from build123d import *

# Parameters (mm, degrees)
SKETCH1_W                 = 33
SKETCH1_H                 = 28
SKETCH1_R                 = 0.75
BOSS_EXTRUDE1_DEPTH       = 1.5
SKETCH2_W                 = 13
SKETCH2_H                 = 10
BOSS_EXTRUDE2_DEPTH       = 6.3
SKETCH3_W                 = 12
SKETCH3_H                 = 5.3
CUT_EXTRUDE1_DEPTH        = 9.5
CUT_EXTRUDE2_REACH        = 25.31
SKETCH5_W                 = 11
SKETCH5_H                 = 2
BOSS_EXTRUDE3_DEPTH       = 9.5
CHAMFER1_SIZE             = 1
CHAMFER1_SIZE2            = 1.804047755
CHAMFER1_OF_MIRROR4_SIZE2 = 1
CHAMFER1_OF_MIRROR4_SIZE  = 1.804047755


with BuildPart() as part:
    # Sketch1 → Boss-Extrude1 (new body)
    with BuildSketch(Plane(origin=(0, 0, 0), x_dir=(1, 0, 0), z_dir=(0, 1, 0))):
        Rectangle(SKETCH1_W, SKETCH1_H)
        with Locations(Location((-13.95, 11.5, 0), (0, 0, 270))):
            Circle(SKETCH1_R, mode=Mode.SUBTRACT)
        with Locations(Location((13.95, 11.5, 0), (0, 0, 270))):
            Circle(SKETCH1_R, mode=Mode.SUBTRACT)
        with Locations(Location((13.95, -1.7, 0), (0, 0, 270))):
            Circle(SKETCH1_R, mode=Mode.SUBTRACT)
        with Locations(Location((-13.95, -1.7, 0), (0, 0, 270))):
            Circle(SKETCH1_R, mode=Mode.SUBTRACT)
    extrude(amount=BOSS_EXTRUDE1_DEPTH)

    # Sketch2 → Boss-Extrude2 (add)
    with BuildSketch(Plane(origin=(0, 1.5, 0), x_dir=(1, 0, 0), z_dir=(0, 1, 0))):
        with Locations((-8.1, -9.5)):
            Rectangle(SKETCH2_W, SKETCH2_H)
    boss_extrude2 = extrude(amount=BOSS_EXTRUDE2_DEPTH)

    # Sketch3 → Cut-Extrude1 (cut)
    with BuildSketch(Plane.XY.offset(14.5)):
        with Locations((-8.1, 4.65)):
            Rectangle(SKETCH3_W, SKETCH3_H)
    cut_extrude1 = extrude(amount=-CUT_EXTRUDE1_DEPTH, mode=Mode.SUBTRACT)

    # Sketch4 → Cut-Extrude2 (cut, up to next)
    with BuildSketch(Plane(origin=(0, 7.8, 0), x_dir=(1, 0, 0), z_dir=(0, 1, 0)), mode=Mode.PRIVATE) as cut_extrude2_sk1:
        with BuildLine():
            Line((-13.614934874, -7.733680754), (-13.022262005, -10.296990911))
            ThreePointArc((-13.022262005, -10.296990911), (-13.006856344, -10.386514555), (-13.001698958, -10.477207547))
            Line((-13.001698958, -10.477207547), (-13.001698958, -11.69747768))
            ThreePointArc((-13.001698958, -11.69747768), (-12.650227096, -12.546005817), (-11.801698958, -12.89747768))
            Line((-11.801698958, -12.89747768), (-10.586140238, -12.89747768))
            ThreePointArc((-10.586140238, -12.89747768), (-9.7376121, -12.546005817), (-9.386140238, -11.69747768))
            Line((-9.386140238, -11.69747768), (-9.386140238, -10.477207547))
            ThreePointArc((-9.386140238, -10.477207547), (-9.380982852, -10.386514555), (-9.365577191, -10.296990911))
            Line((-9.365577191, -10.296990911), (-8.772904322, -7.733680754))
            ThreePointArc((-8.772904322, -7.733680754), (-8.922709401, -7.493767357), (-9.162622799, -7.643572436))
            Line((-9.162622799, -7.643572436), (-9.755295667, -10.206882592))
            ThreePointArc((-9.755295667, -10.206882592), (-9.778404159, -10.34116806), (-9.786140238, -10.477207547))
            Line((-9.786140238, -10.477207547), (-9.786140238, -11.69747768))
            ThreePointArc((-9.786140238, -11.69747768), (-10.020454813, -12.263163104), (-10.586140238, -12.49747768))
            Line((-10.586140238, -12.49747768), (-11.801698958, -12.49747768))
            ThreePointArc((-11.801698958, -12.49747768), (-12.367384383, -12.263163104), (-12.601698958, -11.69747768))
            Line((-12.601698958, -11.69747768), (-12.601698958, -10.477207547))
            ThreePointArc((-12.601698958, -10.477207547), (-12.609435037, -10.34116806), (-12.632543529, -10.206882592))
            Line((-12.632543529, -10.206882592), (-13.225216397, -7.643572436))
            ThreePointArc((-13.225216397, -7.643572436), (-13.465129794, -7.493767357), (-13.614934874, -7.733680754))
        make_face()
    cut_extrude2_tool1 = extrude(cut_extrude2_sk1.sketch, amount=-CUT_EXTRUDE2_REACH, mode=Mode.PRIVATE) & part.part
    # Sketch4 → Cut-Extrude2 (cut, up to next)
    with BuildSketch(Plane(origin=(0, 7.8, 0), x_dir=(1, 0, 0), z_dir=(0, 1, 0)), mode=Mode.PRIVATE) as cut_extrude2_sk2:
        with BuildLine():
            Line((-7.037377201, -7.643572436), (-6.444704333, -10.206882592))
            ThreePointArc((-6.444704333, -10.206882592), (-6.421595841, -10.34116806), (-6.413859762, -10.477207547))
            Line((-6.413859762, -10.477207547), (-6.413859762, -11.69747768))
            ThreePointArc((-6.413859762, -11.69747768), (-6.179545187, -12.263163104), (-5.613859762, -12.49747768))
            Line((-5.613859762, -12.49747768), (-4.398301042, -12.49747768))
            ThreePointArc((-4.398301042, -12.49747768), (-3.832615617, -12.263163104), (-3.598301042, -11.69747768))
            Line((-3.598301042, -11.69747768), (-3.598301042, -10.477207547))
            ThreePointArc((-3.598301042, -10.477207547), (-3.590564963, -10.34116806), (-3.567456471, -10.206882592))
            Line((-3.567456471, -10.206882592), (-2.974783603, -7.643572436))
            ThreePointArc((-2.974783603, -7.643572436), (-2.734870206, -7.493767357), (-2.585065126, -7.733680754))
            Line((-2.585065126, -7.733680754), (-3.177737995, -10.296990911))
            ThreePointArc((-3.177737995, -10.296990911), (-3.193143656, -10.386514555), (-3.198301042, -10.477207547))
            Line((-3.198301042, -10.477207547), (-3.198301042, -11.69747768))
            ThreePointArc((-3.198301042, -11.69747768), (-3.549772904, -12.546005817), (-4.398301042, -12.89747768))
            Line((-4.398301042, -12.89747768), (-5.613859762, -12.89747768))
            ThreePointArc((-5.613859762, -12.89747768), (-6.4623879, -12.546005817), (-6.813859762, -11.69747768))
            Line((-6.813859762, -11.69747768), (-6.813859762, -10.477207547))
            ThreePointArc((-6.813859762, -10.477207547), (-6.819017148, -10.386514555), (-6.834422809, -10.296990911))
            Line((-6.834422809, -10.296990911), (-7.427095678, -7.733680754))
            ThreePointArc((-7.427095678, -7.733680754), (-7.277290599, -7.493767357), (-7.037377201, -7.643572436))
        make_face()
    cut_extrude2_tool2 = extrude(cut_extrude2_sk2.sketch, amount=-CUT_EXTRUDE2_REACH, mode=Mode.PRIVATE) & part.part
    cut_extrude2_1 = cut_extrude2_tool1.solids().sort_by_distance((-13.247802, 7.8, 8.998967))[0]
    add(cut_extrude2_1, mode=Mode.SUBTRACT)
    cut_extrude2_2 = cut_extrude2_tool2.solids().sort_by_distance((-6.741196, 7.8, 11.087343))[0]
    add(cut_extrude2_2, mode=Mode.SUBTRACT)
    cut_extrude2 = cut_extrude2_1 + cut_extrude2_2  # Cut-Extrude2 as one shape, for the pattern or mirror that repeats it

    # Sketch5 → Boss-Extrude3 (add)
    with BuildSketch(Plane.XY.offset(5)):
        with Locations((-8.1, 5.8)):
            Rectangle(SKETCH5_W, SKETCH5_H)
    boss_extrude3 = extrude(amount=BOSS_EXTRUDE3_DEPTH)

    # Chamfer1
    chamfer1_edges = [part.edges().sort_by_distance(p)[0] for p in [
        (-8.1, 6.8, 14.5),
    ]]
    chamfer1_side = [part.faces().sort_by_distance(p)[0] for p in [
        (-8.1, 5.8, 14.5),
    ]]
    chamfer(chamfer1_edges, length=CHAMFER1_SIZE, length2=CHAMFER1_SIZE2, reference=chamfer1_side[0])

    # Mirror4: Boss-Extrude2, Cut-Extrude1, Cut-Extrude2, Boss-Extrude3 across plane
    add(boss_extrude2.mirror(Plane(origin=(0, 0, 0), x_dir=(0, 0, 1), z_dir=(1, 0, 0))))
    add(cut_extrude1.mirror(Plane(origin=(0, 0, 0), x_dir=(0, 0, 1), z_dir=(1, 0, 0))), mode=Mode.SUBTRACT)
    add(cut_extrude2.mirror(Plane(origin=(0, 0, 0), x_dir=(0, 0, 1), z_dir=(1, 0, 0))), mode=Mode.SUBTRACT)
    add(boss_extrude3.mirror(Plane(origin=(0, 0, 0), x_dir=(0, 0, 1), z_dir=(1, 0, 0))))

    # Chamfer1 of Mirror4
    chamfer1_of_mirror4_edges = [part.edges().sort_by_distance(p)[0] for p in [
        (8.1, 6.8, 14.5),
    ]]
    chamfer(chamfer1_of_mirror4_edges, length=CHAMFER1_OF_MIRROR4_SIZE, length2=CHAMFER1_OF_MIRROR4_SIZE2)


solid = part.part
Geometry: final body of the model. Coordinates: model frame, mm. A direction names the side the tool comes from. Give positions to 0.01 mm unless a question says otherwise; leave off trailing zeros. Write each loop counter-clockwise with the first axis right and the second up, starting at its lowest first coordinate (ties: lowest second). Pieces come first, ordered by that corner, then holes. Notation, with made-up numbers: (-21.5, 88.25) - (14.5, 88.25) arc R23 cw to (14.5, 120.25) - close; hole circle Ø7 at (27, -37.75). An arc over 180 degrees is marked (long way). Return JSON: item names as keys, results as strings. Group by question number.
1) Set-up query: faces 4 (the flat face through (8, 2, 10)), 5 (the flat face through (0, 1, 14)), 6 (the flat face through (14.6, 5, 10)), 7 (the cylindrical face through (9.75, 7.55, 12.56)), 8 (the flat face through (-14.6, 5, 10)). Return all of +Z, -Z, +X, -X, +Y, -Y with unobstructed straight access to the full face (end or side cutting, diameter ignored); none if empty.
2) Section D-D on z = 1.7. Return the cut outline in (x, y), plus the area to 3 significant figures.
3) Section C-C on y = 4. Return the cut outline in (x, z).
4) Section A-A on x = 11. Return the cut outline in (y, z).
5) Section B-B on y = 1. Return the cut outline in (x, z), plus the area to 3 significant figures.
6) First-contact query: P1, Ø1, axis at x = 0, z = -8, coming from the +Y side; P2, Ø0.5, axis at y = 7.5, z = 11, coming from the +X side; P3, Ø1, axis at x = 6.5, y = 4, coming from the -Z side. Flat tips, straight axial feed; report the tip coordinate or a pass-through.
7) Line query: line 1 (X direction, y = 4.75, z = 7.5); line 2 (Y direction, x = -8.5, z = 8.25); line 3 (X direction, y = 0.65, z = -11.5). Output: solid intervals per line, ascending.
8) Mould query, pull axis Y, two halves, no side actions, for faces 1 (the flat face through (8, 6.8, 9)), 2 (the cylindrical face through (13.218, 0.74, 1.537)), 3 (the flat face through (0, 1.5, -3)). Classes: released by +Y, released by -Y, zero draft, split by the parting line, or undercut.
Filled in:
{
 "1": {"face 4": "+Z", "face 5": "+Z, +X, -X, -Y", "face 6": "+Z, -Z, +X, +Y", "face 7": "+Y", "face 8": "+Z, -Z, -X, +Y"},
 "2": {"outline": "(-16.5, 0) - (-14.7, 0) - (-14.7, 1.5) - (-16.5, 1.5) - close; (-13.2, 0) - (13.2, 0) - (13.2, 1.5) - (-13.2, 1.5) - close; (14.7, 0) - (16.5, 0) - (16.5, 1.5) - (14.7, 1.5) - close", "area": "45.0 mm^2"},
 "3": {"outline": "(-14.6, 4.5) - (-1.6, 4.5) - (-1.6, 14.5) - (-2.1, 14.5) - (-2.1, 5) - (-14.1, 5) - (-14.1, 14.5) - (-14.6, 14.5) - close; (1.6, 4.5) - (14.6, 4.5) - (14.6, 14.5) - (14.1, 14.5) - (14.1, 5) - (2.1, 5) - (2.1, 14.5) - (1.6, 14.5) - close"},
 "4": {"outline": "(0, -14) - (1.5, -14) - (1.5, 4.5) - (7.8, 4.5) - (7.8, 12.5) - (7.3, 12.5) - (7.3, 5) - (6.8, 5) - (6.8, 12.7) - (5.8, 14.5) - (4.8, 14.5) - (4.8, 5) - (2, 5) - (2, 14.5) - (1.5, 14.5) - (1.5, 14) - (0, 14) - close; (7.3, 12.9) - (7.8, 12.9) - (7.8, 14.5) - (7.3, 14.5) - close"},
 "5": {"outline": "(-16.5, -14) - (16.5, -14) - (16.5, 14) - (-16.5, 14) - close; hole circle Ø1.5 at (-13.95, -11.5); hole circle Ø1.5 at (-13.95, 1.7); hole circle Ø1.5 at (13.95, -11.5); hole circle Ø1.5 at (13.95, 1.7)", "area": "917 mm^2"},
 "6": {"P1": "stops at y = 1.5", "P2": "stops at x = 14.6", "P3": "stops at z = 4.5"},
 "7": {"line 1": "x = -14.6 to -14.1, -2.1 to -1.6, 1.6 to 2.1, 14.1 to 14.6", "line 2": "y = 0 to 2, 4.8 to 6.8, 7.3 to 7.8", "line 3": "x = -16.5 to -14.7, -13.2 to 13.2, 14.7 to 16.5"},
 "8": {"face 1": "undercut", "face 2": "zero draft", "face 3": "released by +Y"}
}
